Design review of the part built by this model. Coordinates are the model's own, in mm. Face numbers are marked on the shaded views. A direction names the side the tool comes from. Give positions to 0.01 mm unless a question says otherwise; leave off trailing zeros. Write each loop counter-clockwise with the first axis right and the second up, starting at its lowest first coordinate (ties: lowest second). Pieces come first, ordered by that corner, then holes. Notation, with made-up numbers: M 12.25,35.25 L 36.25,35.25 A17 ccw 36.25,64.25 Z; hole C 26,2.5 d6. An arc over 180 degrees is marked long. Write each question's results on one line, items separated by ' | '. Start each with the question number.
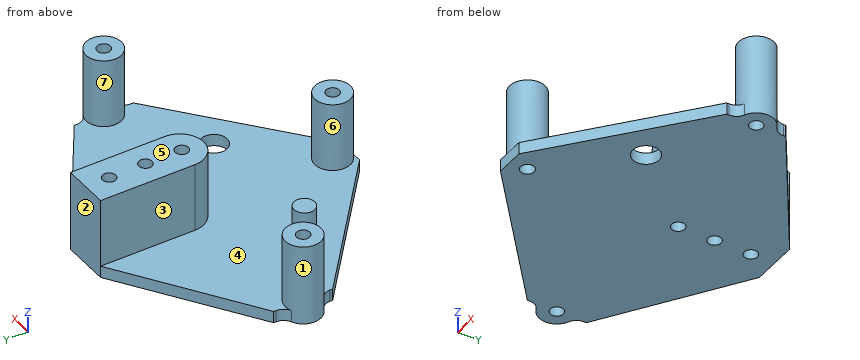
from build123d import *

# Parameters (mm, degrees)
SKETCH1_W               = 84.00796
SKETCH1_H               = 71.2724
BOSS_EXTRUDE1_DEPTH     = 3.175
SKETCH5_R               = 4.7625
BOSS_EXTRUDE3_DEPTH     = 3.175
SKETCH3_R               = 1.8415
CUT_EXTRUDE1_DEPTH      = 114.886040389
BOSS_EXTRUDE4_START     = 18.542
SKETCH6_R               = 4.7625
BOSS_EXTRUDE4_DEPTH     = 18.542
CUT_EXTRUDE2_DEPTH      = 116.341906237
CUT_EXTRUDE2_DEPTH_BACK = 116.341906237
SKETCH4_R               = 1.778
SKETCH7_R               = 1.778
CUT_EXTRUDE3_DEPTH      = 116.894683482
SKETCH8_R               = 3.556
SKETCH8_R_2             = 1.905
CUT_EXTRUDE4_DEPTH      = 116.894683482
CUT_EXTRUDE5_DEPTH      = 116.894683482
FILLET1_R               = 3.175
SKETCH10_R              = 2.794
BOSS_EXTRUDE5_DEPTH     = 6.35
BOSS_EXTRUDE6_START     = 3.175
SKETCH11_R              = 1.905
BOSS_EXTRUDE6_DEPTH     = 3.175


with BuildPart() as part:
    # Sketch1 → Boss-Extrude1 (new body)
    with BuildSketch(Plane.XY):
        with Locations((42.00398, 35.6362)):
            Rectangle(SKETCH1_W, SKETCH1_H)
    extrude(amount=BOSS_EXTRUDE1_DEPTH)

    # Sketch5 → Boss-Extrude3 (add)
    with BuildSketch(Plane.XY.offset(3.175)):
        with Locations((84.00796, 39.524999944)):
            Circle(SKETCH5_R)
        with Locations((0, 39.524999944)):
            Circle(SKETCH5_R)
    extrude(amount=-BOSS_EXTRUDE3_DEPTH)

    # Sketch3 → Cut-Extrude1 (cut, through all)
    with BuildSketch(Plane.XY.offset(3.175)):
        with Locations((42.00398, 4.7625)):
            Circle(SKETCH3_R)
    extrude(amount=-CUT_EXTRUDE1_DEPTH, mode=Mode.SUBTRACT)

    # Sketch6 → Boss-Extrude4 (add)
    with BuildSketch(Plane.XY.offset(3.175).offset(BOSS_EXTRUDE4_START)):
        with Locations((84.00796, 39.524999944)):
            Circle(SKETCH6_R)
        with Locations((0, 39.524999944)):
            Circle(SKETCH6_R)
        with Locations(Location((42.00398, 4.7625, 0), (0, 0, 270))):
            Circle(SKETCH6_R)
        with BuildLine():
            Line((35.65398, 71.2724), (48.35398, 71.2724))
            Line((48.35398, 71.2724), (48.35398, 45.8724))
            ThreePointArc((48.35398, 45.8724), (42.00398, 39.5224), (35.65398, 45.8724))
            Line((35.65398, 45.8724), (35.65398, 71.2724))
        make_face()
    extrude(amount=-BOSS_EXTRUDE4_DEPTH)

    # Sketch4 → Cut-Extrude2 (cut, two sides: drawn at the far end of the back side and taken through both)
    with BuildSketch(Plane.XY.offset(3.175).offset(-CUT_EXTRUDE2_DEPTH_BACK)):
        with Locations((42.00398, 64.9224)):
            Circle(SKETCH4_R)
        with Locations((42.00398, 55.1434)):
            Circle(SKETCH4_R)
        with Locations((42.00398, 45.3644)):
            Circle(SKETCH4_R)
    extrude(amount=CUT_EXTRUDE2_DEPTH + CUT_EXTRUDE2_DEPTH_BACK, mode=Mode.SUBTRACT)

    # Sketch7 → Cut-Extrude3 (cut, through all)
    with BuildSketch(Plane(origin=(0, 0, 0), x_dir=(-1, 0, 0), z_dir=(0, 0, -1))):
        with Locations((-42.00398, 4.7625)):
            Circle(SKETCH7_R)
        with Locations((0, 39.524999944)):
            Circle(SKETCH7_R)
        with Locations((-84.00796, 39.524999944)):
            Circle(SKETCH7_R)
    extrude(amount=-CUT_EXTRUDE3_DEPTH, mode=Mode.SUBTRACT)

    # Sketch8 → Cut-Extrude4 (cut, through all)
    with BuildSketch(Plane(origin=(0, 0, 0), x_dir=(-1, 0, 0), z_dir=(0, 0, -1))):
        with Locations((-61.05398, 24.524999972)):
            Circle(SKETCH8_R)
        with Locations((-22.95398, 24.524999972)):
            Circle(SKETCH8_R_2)
    extrude(amount=-CUT_EXTRUDE4_DEPTH, mode=Mode.SUBTRACT)

    # Sketch9 → Cut-Extrude5 (cut, through all)
    with BuildSketch(Plane(origin=(0, 0, 0), x_dir=(-1, 0, 0), z_dir=(0, 0, -1))):
        Polygon((-84.00796, 0), (-84.00796, 31.587499944), (-45.90796, 0), align=None)
        Polygon((-84.00796, 71.2724), (-84.00796, 47.462499944), (-48.35398, 71.2724), align=None)
    cut_extrude5 = extrude(amount=-CUT_EXTRUDE5_DEPTH, mode=Mode.SUBTRACT)

    # Mirror1: Cut-Extrude5 across plane
    add(cut_extrude5.mirror(Plane(origin=(42.00398, 0, 0), x_dir=(0, 0, 1), z_dir=(1, 0, 0))), mode=Mode.SUBTRACT)

    # Fillet1
    # the kernel refuses this fillet: 3.175 mm, written as the material it adds along each edge
    with BuildSketch(Plane(origin=(84.00796, 34.762499944, 0), x_dir=(0.9789063129307042, 0.2043096436892158, 0), z_dir=(0, 0, 1))) as fillet1_piece_1:
        with BuildLine():
            CenterArc((2.594732475, -3.108027544), FILLET1_R, 101.789089239, 66.421821522)
            Line((-0.513295069, -2.459344425), (0, 0))
            ThreePointArc((0, 0), (0.973024678, -0.100458685), (1.946049356, 0))
        make_face()
    extrude(amount=3.175)
    with BuildSketch(Plane(origin=(84.00796, 44.287499944, 0), x_dir=(0, 1, 0), z_dir=(0, 0, 1)), Plane(origin=(0, 34.762499944, 0), x_dir=(0, -1, 0), z_dir=(0, 0, 1))) as fillet1_piece_2:
        with BuildLine():
            CenterArc((2.512338916, -3.175), FILLET1_R, 90, 66.421821522)
            ThreePointArc((-0.397596651, -1.905), (-0.100458685, -0.973024678), (0, 0))
            Line((0, 0), (2.512338916, 0))
        make_face()
    extrude(amount=3.175)
    with BuildSketch(Plane(origin=(0, 44.287499944, 0), x_dir=(0, 1, 0), z_dir=(0, 0, 1))) as fillet1_piece_3:
        with BuildLine():
            CenterArc((2.512338916, 3.175), FILLET1_R, 203.578178478, 66.421821522)
            ThreePointArc((-0.397596651, 1.905), (-0.100458685, 0.973024678), (0, 0))
            Line((0, 0), (2.512338916, 0))
        make_face()
    extrude(amount=3.175)

    # Sketch10 → Boss-Extrude5 (add)
    with BuildSketch(Plane.XY.offset(3.175)):
        with Locations(Location((22.95398, 24.524999972, 0), (0, 0, 180))):
            Circle(SKETCH10_R)
    extrude(amount=BOSS_EXTRUDE5_DEPTH)

    # Sketch11 → Boss-Extrude6 (add)
    with BuildSketch(Plane(origin=(0, 0, 3.175), x_dir=(-1, 0, 0), z_dir=(0, 0, -1)).offset(BOSS_EXTRUDE6_START)):
        with Locations((-22.95398, 24.524999972)):
            Circle(SKETCH11_R)
    extrude(amount=-BOSS_EXTRUDE6_DEPTH)


solid = part.part
Q1. We need section A-A on z = 13.75. Count the separate pieces of the cut face and the enclosed holes in it, and give its area (3 significant figures).
Q2. We need section B-B on y = 58.5. Write out the cut boundary in (x, z) (3 decimals).
Q3. We need section C-C on x = 51. Write out the cut boundary in (y, z) (3 decimals), and give its area (3 significant figures).
Q4. For pin 1 Ø3 at (x, y) = (84.01, 39.52) entering from +Z; pin 2 Ø0.5 at (y, z) = (47, 1) entering from +X; pin 3 Ø12 at (y, z) = (58.5, 13.5) entering from +X; pin 4 Ø0.7 at (y, z) = (32, 1.5) entering from -X, all flat-tipped, find the tip position at first contact; note any pin that passes through.
Q5. For the marked faces 1, 2 and 3, list the 3-axis set-ups (+Z, -Z, +X, -X, +Y, -Y) from which the entire face can be reached by the end or side of a thin tool; tool diameter is ignored.
Q6. We need section D-D on y = 49.5. Write out the cut boundary in (x, z) (3 decimals).
Q7. The part is to be moulded in two halves that separate along X. For the marked faces 4, 5, 6 and 7, say which applies: pulls with the +X half, pulls with the -X half, needs draft (parallel to the pull), parting line crosses it, or undercut.
Q8. Wall thickness on line 1 along Y through (x, z) = (0, 16.75); line 2 along X through (y, z) = (55, 3.5); line 3 along X through (y, z) = (45.5, 10.5): over which ranges is each line inside the solid? List them lowest first. Write a range as from..to.
Answer sheet:
1) separate pieces: 4 | enclosed holes: 6 | area: 540 mm^2
2) outline: M 16.528,0 L 67.48,0 L 67.48,3.175 L 48.354,3.175 L 48.354,21.717 L 35.654,21.717 L 35.654,3.175 L 16.528,3.175 Z
3) outline: M 4.222,0 L 69.505,0 L 69.505,3.175 L 4.222,3.175 Z | area: 207 mm^2
4) pin 1: through | pin 2: x = 84.01 | pin 3: x = 48.35 | pin 4: x = 0
5) face 1: +Z | face 2: +Z, -Z, +X, -X, +Y | face 3: +Z, -X, +Y, -Y
6) outline: M 3.051,0 L 80.957,0 L 80.957,3.175 L 48.354,3.175 L 48.354,21.717 L 35.654,21.717 L 35.654,3.175 L 3.051,3.175 Z
7) face 4: undercut | face 5: needs draft | face 6: parting line crosses it | face 7: undercut
8) line 1: 34.76..37.75, 41.3..44.29 | line 2: 35.65..40.23, 43.78..48.35 | line 3: 35.66..40.23, 43.78..48.34
